Input: part model. Units: mm. Frame: model coordinates. A direction names the side the tool comes from. Give positions to 0.01 mm unless a question says otherwise; leave off trailing zeros. Order: outer loops, then holes, each group sorted by start corner. A loop starts at its lowest first (then second) coordinate and runs counter-clockwise, first axis right, second up.
Autodesk Fusion 360 part; units mm, degrees
sketch "Sketch1" plane through (0, 0, 0) normal (0, 0, 1) x (1, 0, 0)
  circle A0 centre (0, 0) radius 25
  circle A1 centre (0, 0) radius 29
  dimension "d3" = 50
  dimension "d4" = 4
extrude "Extrude1" add sketch "Sketch1" along normal blind 200 contours A0 makes body 1
extrude "Extrude2" add sketch "Sketch1" against normal blind 30 separate body makes body 2
extrude "Extrude3" add sketch "Sketch1" against normal blind 15 contours A0 bodies 1 2
sketch "Sketch2" plane through (0, 0, 200) normal (0, 0, 1) x (1, 0, 0)
  circle A0 centre (0, 0) radius 25
  circle A1 centre (0, 0) radius 29
  dimension "d9" = 4
extrude "Extrude4" add sketch "Sketch2" along normal blind 15 contours A0 bodies 1
extrude "Extrude5" add sketch "Sketch2" along normal blind 30 bodies 1
1) Cut plane C-C (z = 132.5). Return the cut outline in (x, y), then the cut area to 3 significant figures.
2) Line query: probe 1 along Z at (x, y) = (9, 24.5); probe 2 along Z at (x, y) = (-0.5, 18); probe 3 along Y at (x, z) = (0, 224.5). Output: solid intervals per line, ascending.
3) First-contact query: P1, Ø1, axis at x = 14.5, z = 84, coming from the +Y side; P2, Ø12, axis at x = 15, y = -10.5, coming from the +Z side; P3, Ø1, axis at y = 9.5, z = 162, coming from the +X side. Flat tips, straight axial feed; report the tip coordinate or a pass-through.
4) Cut plane A-A (y = 0). Return the cut outline in (x, z).
5) Pull-direction query (Y, two-part tool) for faces 1 (the face through (23.846, -7.509, 98.6)), 2 (the face through (0, 0, -15)), 3 (the face through (13, 22, 230)); classes: pulls with the +Y half, pulls with the -Y half, needs draft (parallel to the pull), parting line crosses it, or undercut.
6) Reachability of faces 4 (the face through (13, 22, -30)), 5 (the face through (13, 22, 200)), 6 (the face through (23.846, 7.509, -22.395)), 7 (the face through (0, 0, 215)), 8 (the face through (13.38, -25.73, -14.79)) from +Z, -Z, +X, -X, +Y, -Y: full face, straight path, thin tool, end or side. Return the list, or none.
Geometry says:
1. outline: circle Ø50 at (0, 0)
1. area: 1,960 mm2
2. probe 1: z = -30 to 0, 200 to 230
2. probe 2: z = -15 to 215
2. probe 3: y = -29 to -25, 25 to 29
3. P1: stops at y = 20.71
3. P2: stops at z = 215
3. P3: stops at x = 23.32
4. outline: (-29, -30) - (-25, -30) - (-25, -15) - (25, -15) - (25, -30) - (29, -30) - (29, 0) - (25, 0) - (25, 200) - (29, 200) - (29, 230) - (25, 230) - (25, 215) - (-25, 215) - (-25, 230) - (-29, 230) - (-29, 200) - (-25, 200) - (-25, 0) - (-29, 0) - close
5. face 1: parting line crosses it
5. face 2: undercut
5. face 3: needs draft
6. face 4: -Z, +X, -X, +Y, -Y
6. face 5: none
6. face 6: -Z
6. face 7: +Z
6. face 8: +Z, -Z
